Model file for the job. Use its own axes, mm. Face numbers are marked on the shaded views. A direction names the side the tool comes from. Round coordinates to 2 decimals unless told otherwise and drop trailing zeros. Loops run counter-clockwise (first coordinate to the right, second up) from the corner with the lowest first, then second, coordinate; pieces in that order, holes last. Notation, with made-up numbers: (-6, -36) -> (1, -36) arc R22 cw to (1, -20) -> close; hole circle Ø6 at (24, 40). An arc over 180 degrees is marked (long way). Use a Markdown table: item, result.
from build123d import *

# Parameters (mm, degrees)
F0_R     = 4
F0_R_2   = 2.4
F0_R_3   = 1.6
F1_DEPTH = 9.6
F2_DEPTH = 11.2
F3_DEPTH = 8
F4_R     = 4
F4_R_2   = 3.2568542495
F5_DEPTH = 1.5999999596


with BuildPart() as f1:
    # F0 (on Top) → F1 (new body)
    with BuildSketch(Plane.XY):
        Circle(F0_R)
        Circle(F0_R_2, mode=Mode.SUBTRACT)
        Circle(F0_R_2)
        Circle(F0_R_3, mode=Mode.SUBTRACT)
    extrude(amount=F1_DEPTH)

    # F0 (on Top) → F2 (join)
    with BuildSketch(Plane.XY):
        Circle(F0_R_2)
        Circle(F0_R_3, mode=Mode.SUBTRACT)
    extrude(amount=F2_DEPTH)

    # F0 (on Top) → F3 (cut, through all)
    with BuildSketch(Plane.XY):
        Circle(F0_R_2)
        Circle(F0_R_3, mode=Mode.SUBTRACT)
    extrude(amount=F3_DEPTH, mode=Mode.SUBTRACT)

    # F4 (on Top) → F5 (cut)
    with BuildSketch(Plane.XY):
        Circle(F4_R)
        Circle(F4_R_2, mode=Mode.SUBTRACT)
    extrude(amount=F5_DEPTH, mode=Mode.SUBTRACT)


solid = f1.part
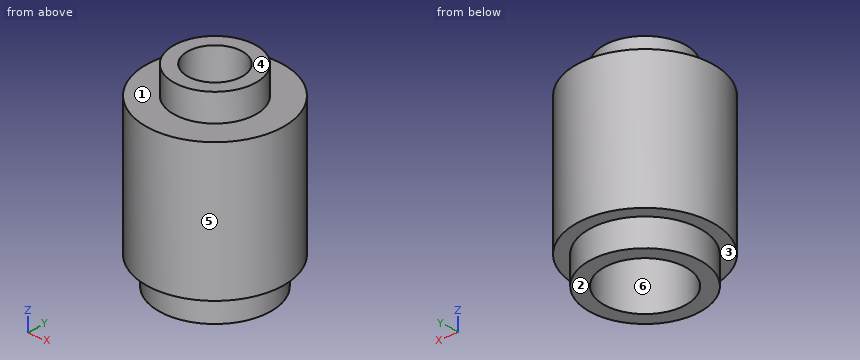
Q1. Flat gauge pin, fed straight in: pin 1 (2.5 mm diameter, centred on x = 0, y = 1, fed in from -Z). Where does the tip first touch, or does it go through?
Results list:
| item | result |
|---|---|
| pin 1 | stops at z = 8 |
Q2. Tool access for the marked faces 1, 2 and 3: list every direction of +Z, -Z, +X, -X, +Y, -Y with a clear straight run to the whole face (end or side of a thin tool).
Results list:
| item | result |
|---|---|
| face 1 | +Z |
| face 2 | -Z, +X, -X, +Y, -Y |
| face 3 | -Z |
Q3. Drill centre lines: L1, parallel to Y at x = 0, z = 9.1; L2, parallel to Y at x = 0, z = 9.9; L3, parallel to Z at x = 2.5, y = -0.75. Where is each one in solid material? Low to high. Write a range as from..to.
Results list:
| item | result |
|---|---|
| L1 | y = -4..-1.6, 1.6..4 |
| L2 | y = -2.4..-1.6, 1.6..2.4 |
| L3 | z = 0..9.6 |
Q4. Band-saw the part on D-D, the plane x = 1.75. Give the cut face in (y, z).
Results list:
| item | result |
|---|---|
| outline | (-3.6, 1.6) -> (-2.75, 1.6) -> (-2.75, 0) -> (-1.64, 0) -> (-1.64, 8) -> (1.64, 8) -> (1.64, 0) -> (2.75, 0) -> (2.75, 1.6) -> (3.6, 1.6) -> (3.6, 9.6) -> (1.64, 9.6) -> (1.64, 11.2) -> (-1.64, 11.2) -> (-1.64, 9.6) -> (-3.6, 9.6) -> close |
Q5. Band-saw the part on C-C, the plane z = 10. Give the cut face in (x, y).
Results list:
| item | result |
|---|---|
| outline | circle Ø4.8 at (0, 0); hole circle Ø3.2 at (0, 0) |
Q6. Pull direction Y, two halves, no side cores. Call the marked faces 4, 5 and 6: released by +Y, released by -Y, zero draft, split by the parting line, or undercut.
Results list:
| item | result |
|---|---|
| face 4 | zero draft |
| face 5 | split by the parting line |
| face 6 | undercut |
Q7. Band-saw the part on A-A, the plane x = 0. Give the cut face in (y, z).
Results list:
| item | result |
|---|---|
| outline | (-4, 1.6) -> (-3.26, 1.6) -> (-3.26, 0) -> (-2.4, 0) -> (-2.4, 8) -> (-1.6, 8) -> (-1.6, 11.2) -> (-2.4, 11.2) -> (-2.4, 9.6) -> (-4, 9.6) -> close; (1.6, 8) -> (2.4, 8) -> (2.4, 0) -> (3.26, 0) -> (3.26, 1.6) -> (4, 1.6) -> (4, 9.6) -> (2.4, 9.6) -> (2.4, 11.2) -> (1.6, 11.2) -> close |
